Part model, mm, in its own coordinate system. A direction names the side the tool comes from. Give positions to 0.01 mm unless a question says otherwise; leave off trailing zeros. Order: outer loops, then holes, each group sorted by start corner. A loop starts at its lowest first (then second) coordinate and runs counter-clockwise, first axis right, second up. Notation, with made-up numbers: M 56,26 L 103,26 A8 cw 103,30 Z; hole C 1,28 d8. An arc over 180 degrees is marked long. Write each question's results on one line, items separated by ' | '. Start each with the question number.
from build123d import *

# Parameters (mm, degrees)
ESQUISSE1_W        = 45
ESQUISSE1_H        = 42
ESQUISSE1_R        = 1.75
ESQUISSE1_R_2      = 11.125
BOSS_EXTRU_1_DEPTH = 3
ESQUISSE3_W        = 45
ESQUISSE3_H        = 20
ESQUISSE3_R        = 1
BOSS_EXTRU_2_DEPTH = 3


with BuildPart() as part:
    # Esquisse1 → Boss.-Extru.1 (new body)
    with BuildSketch(Plane.XY):
        with Locations((15.5, 15)):
            Rectangle(ESQUISSE1_W, ESQUISSE1_H)
        with Locations((0, 31)):
            Circle(ESQUISSE1_R, mode=Mode.SUBTRACT)
        with Locations((31, 31)):
            Circle(ESQUISSE1_R, mode=Mode.SUBTRACT)
        with Locations((31, 0)):
            Circle(ESQUISSE1_R, mode=Mode.SUBTRACT)
        Circle(ESQUISSE1_R, mode=Mode.SUBTRACT)
        with Locations((15.5, 15.5)):
            Circle(ESQUISSE1_R_2, mode=Mode.SUBTRACT)
    extrude(amount=BOSS_EXTRU_1_DEPTH)

    # Esquisse3 → Boss.-Extru.2 (add)
    with BuildSketch(Plane.XZ.offset(6)):
        with Locations((15.5, 10)):
            Rectangle(ESQUISSE3_W, ESQUISSE3_H)
        with Locations((-4.5, 5)):
            Circle(ESQUISSE3_R, mode=Mode.SUBTRACT)
        with Locations(Location((35.5, 5, 0), (0, 0, 180))):
            Circle(ESQUISSE3_R, mode=Mode.SUBTRACT)
    extrude(amount=BOSS_EXTRU_2_DEPTH)


solid = part.part
(1) Tool access for faces 4 (the cylindrical face through (1.617, -0.67, 1.479)), 5 (the flat face through (15, -6, 12)): list every direction of +Z, -Z, +X, -X, +Y, -Y with a clear straight run to the whole face (end or side of a thin tool).
(2) Pull direction X, two halves, no side cores. Call faces 1 (the cylindrical face through (25.777, 11.239, 1.479)), 2 (the flat face through (15, -9, 10)), 3 (the flat face through (-7, 8.6, 2.5)): +X half, -X half, draft (parallel to the pull), parting line (faces both ways), or undercut.
(3) Saw through at B-B on x = -4.5. Give the cut face in (y, z), plus the area to 3 significant figures.
(4) Saw through at A-A on x = 0. Give the cut face in (y, z).
(5) Probe L1, parallel to Y at x = 0, z = 1.1; L2, parallel to Y at x = -1, z = 1.75; L3, parallel to Y at x = 7, z = 18.25. List the from-to ranges inside material, lowest first.
(6) Saw through at D-D on x = 15.5. Give the cut face in (y, z) (3 decimals).
(7) Saw through at C-C on y = 31. Give the cut face in (x, z), plus the area to 3 significant figures.
(8) Drop flat-ended pins along their axis: P1, Ø1, axis at x = 5.5, y = 3.5, coming from the +Z side; P2, Ø5, axis at x = 20, z = 11, coming from the +Y side; P3, Ø1.2, axis at x = 35.5, z = 5, coming from the -Y side. Give the stop position or say it passes through.
Taken from the geometry:
1) face 4: +Z, -Z | face 5: +Z, +X, -X, +Y
2) face 1: undercut | face 2: draft | face 3: -X half
3) outline: M -9,0 L 36,0 L 36,3 L -6,3 L -6,4 L -9,4 Z; M -9,6 L -6,6 L -6,20 L -9,20 Z | area: 180 mm²
4) outline: M -9,0 L -1.75,0 L -1.75,3 L -6,3 L -6,20 L -9,20 Z; M 1.75,0 L 29.25,0 L 29.25,3 L 1.75,3 Z; M 32.75,0 L 36,0 L 36,3 L 32.75,3 Z
5) L1: y = -9 to -1.75, 1.75 to 29.25, 32.75 to 36 | L2: y = -9 to -1.44, 1.44 to 29.56, 32.44 to 36 | L3: y = -9 to -6
6) outline: M -9,0 L 4.375,0 L 4.375,3 L -6,3 L -6,20 L -9,20 Z; M 26.625,0 L 36,0 L 36,3 L 26.625,3 Z
7) outline: M -7,0 L -1.75,0 L -1.75,3 L -7,3 Z; M 1.75,0 L 29.25,0 L 29.25,3 L 1.75,3 Z; M 32.75,0 L 38,0 L 38,3 L 32.75,3 Z | area: 114 mm²
8) P1: stops at z = 3 | P2: stops at y = -6 | P3: passes through
